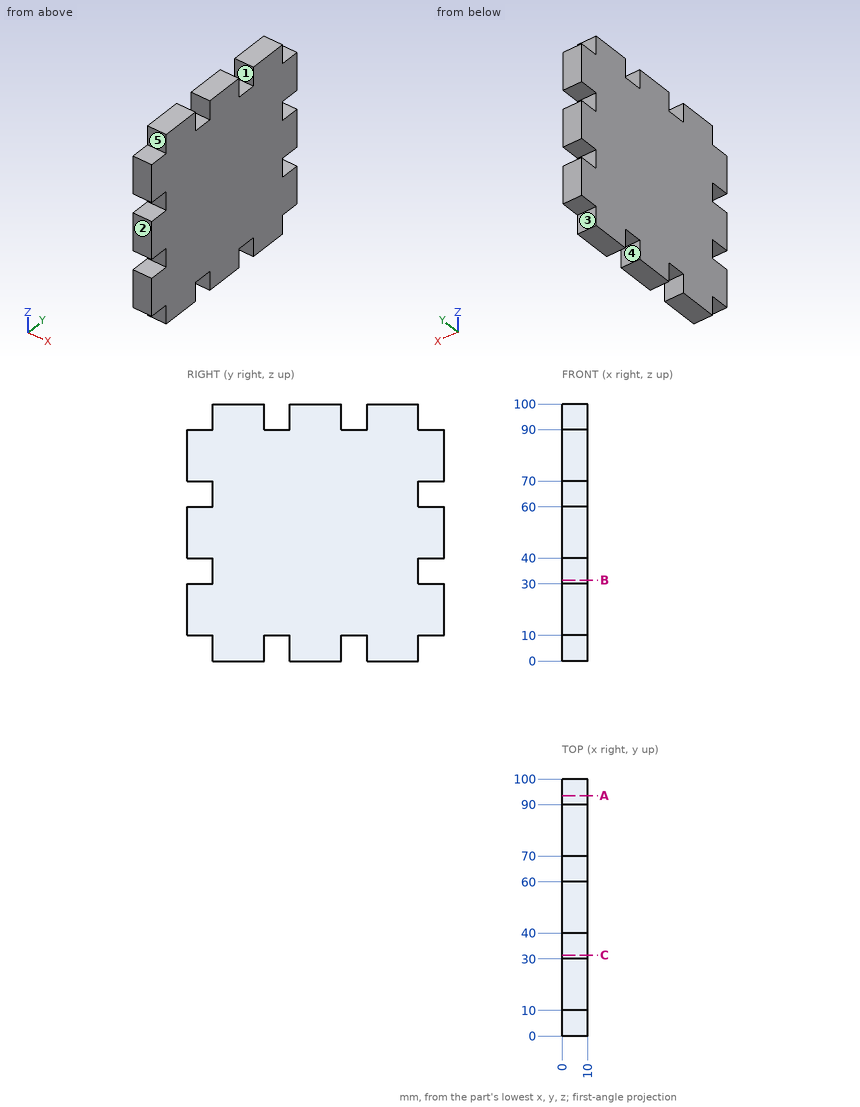
Verification items for this drawing (mm, ordinates from the low corner). A direction names the side the tool comes from. Coordinates: 2 decimals unless noted, no trailing zeros. Order: outer loops, then holes, each group sorted by start corner. A loop starts at its lowest first (then second) coordinate and runs counter-clockwise, first axis right, second up. Notation, with made-up numbers: (-0.75, 10) - (13.25, 10) arc R26 cw to (13.25, 33) - close; hole circle Ø3 at (12.25, 16). An arc over 180 degrees is marked (long way). Answer in a Markdown table with one row per item. Add a question column.
1. Section check B-B (z = 31.5). Enter the section's corners in (x, y).
2. Material ranges on L1, parallel to Y at x = 9.75, z = 8; L2, parallel to Z at x = 7.5, y = 61.5, recorded low to high. Write a range as [from, to].
3. Access from +Z, -Z, +X, -X, +Y, -Y to the whole of each face (thin tool, end or side, straight path). Record for the marked faces 1, 2, 3, 4 and 5.
4. Section check A-A (y = 93.5). Enter the section's corners in (x, z), plus the area to 3 significant figures.
5. Gauge pin test, flat ends, axial feed: pin 1 Ø4 at (x, z) = (1.5, 37.5) entering from +Y; pin 2 Ø3 at (x, z) = (4.5, 95.5) entering from -Y; pin 3 Ø1.5 at (x, y) = (4, 35.5) entering from +Z. Record the tip position at first contact, or that the pin passes through.
Data:
| question | item | result |
|---|---|---|
| 1 | outline | (0, 10) - (10, 10) - (10, 90) - (0, 90) - close |
| 2 | L1 | y = [10, 30], [40, 60], [70, 90] |
| 2 | L2 | z = [10, 90] |
| 3 | face 1 | +Z, +X, -X |
| 3 | face 2 | +Z, -Z, +X, -X, -Y |
| 3 | face 3 | -Z, +X, -X, +Y |
| 3 | face 4 | -Z, +X, -X |
| 3 | face 5 | +Z, +X, -X, -Y |
| 4 | outline | (0, 10) - (10, 10) - (10, 30) - (0, 30) - close; (0, 40) - (10, 40) - (10, 60) - (0, 60) - close; (0, 70) - (10, 70) - (10, 90) - (0, 90) - close |
| 4 | area | 600 mm² |
| 5 | pin 1 | stops at y = 90 |
| 5 | pin 2 | stops at y = 10 |
| 5 | pin 3 | stops at z = 90 |
